from build123d import *

# Parameters (mm, degrees)
SKETCH1_R           = 56.515
BOSS_EXTRUDE1_DEPTH = 19.05


with BuildPart() as part:
    # Sketch1 → Boss-Extrude1 (new body)
    # profile 1 of 6: a face of its own
    with BuildSketch(Plane.XY):
        Polygon((-263.964543073, 0), (-131.982271537, 228.6), (0, 0), align=None)
        with Locations(Location((-131.982271537, 76.2, 0), (0, 0, 180))):
            Circle(SKETCH1_R, mode=Mode.SUBTRACT)
    # profile 2 of 6: a face of its own
    with BuildSketch(Plane.XY):
        Polygon((131.982271537, 228.6), (0, 0), (-131.982271537, 228.6), align=None)
        with Locations(Location((0, 152.4, 0), (0, 0, 180))):
            Circle(SKETCH1_R, mode=Mode.SUBTRACT)
    # profile 3 of 6: a face of its own
    with BuildSketch(Plane.XY):
        Polygon((263.964543073, 0), (0, 0), (131.982271537, 228.6), align=None)
        with Locations(Location((131.982271537, 76.2, 0), (0, 0, 180))):
            Circle(SKETCH1_R, mode=Mode.SUBTRACT)
    # profile 4 of 6: a face of its own
    with BuildSketch(Plane.XY):
        Polygon((131.982271537, -228.6), (0, 0), (263.964543073, 0), align=None)
        with Locations(Location((131.982271537, -76.2, 0), (0, 0, 180))):
            Circle(SKETCH1_R, mode=Mode.SUBTRACT)
    # profile 5 of 6: a face of its own
    with BuildSketch(Plane.XY):
        Polygon((-131.982271537, -228.6), (0, 0), (131.982271537, -228.6), align=None)
        with Locations(Location((0, -152.4, 0), (0, 0, 180))):
            Circle(SKETCH1_R, mode=Mode.SUBTRACT)
    # profile 6 of 6: a face of its own
    with BuildSketch(Plane.XY):
        Polygon((-263.964543073, 0), (0, 0), (-131.982271537, -228.6), align=None)
        with Locations(Location((-131.982271537, -76.2, 0), (0, 0, 180))):
            Circle(SKETCH1_R, mode=Mode.SUBTRACT)
    extrude(amount=BOSS_EXTRUDE1_DEPTH)


solid = part.part
Part model, mm, in its own coordinate system. Coordinates: 2 decimals unless noted, no trailing zeros. Order: outer loops, then holes, each group sorted by start corner. A loop starts at its lowest first (then second) coordinate and runs counter-clockwise, first axis right, second up. Notation, with made-up numbers: M 20.5,61 L 38.5,61 A20 cw 38.5,84 Z; hole C 0,3 d11. An arc over 180 degrees is marked long. Use a Markdown table: item, result.
(1) Cut at A-A on x = 0. Write the cut outline in (y, z) (3 decimals).
A:
| item | result |
|---|---|
| outline | M -228.6,0 L -208.915,0 L -208.915,19.05 L -228.6,19.05 Z; M -95.885,0 L 95.885,0 L 95.885,19.05 L -95.885,19.05 Z; M 208.915,0 L 228.6,0 L 228.6,19.05 L 208.915,19.05 Z |
(2) Cut at C-C on y = 83. Write the cut outline in (x, z).
A:
| item | result |
|---|---|
| outline | M -216.04,0 L -188.09,0 L -188.09,19.05 L -216.04,19.05 Z; M -75.88,0 L 75.88,0 L 75.88,19.05 L -75.88,19.05 Z; M 188.09,0 L 216.04,0 L 216.04,19.05 L 188.09,19.05 Z |
(3) Pull direction Y, two halves, no side cores. Call faces 1 (the flat face through (-2, 228.6, 9)), 2 (the cylindrical face through (12.25, 207.57, 9.39)), 3 (the flat face through (4, 3, 19.05)): released by +Y, released by -Y, zero draft, split by the parting line, or undercut.
A:
| item | result |
|---|---|
| face 1 | released by +Y |
| face 2 | undercut |
| face 3 | zero draft |
(4) Probe L1, parallel to Y at x = 0, z = 13 (3 decimals); L2, parallel to X at y = 93, z = 13; L3, parallel to X at y = -93.5, z = 7.5. List the from-to ranges inside material, lowest first.
A:
| item | result |
|---|---|
| L1 | y = -228.6 to -208.915, -95.885 to 95.885, 208.915 to 228.6 |
| L2 | x = -210.27 to -185.94, -78.02 to 78.02, 185.94 to 210.27 |
| L3 | x = -209.98 to -185.78, -78.18 to 78.18, 185.78 to 209.98 |
(5) Cut at B-B on z = 11. Write the cut outline in (x, y) (3 decimals), then the cut area to 3 significant figures.
A:
| item | result |
|---|---|
| outline | M -263.965,0 L -131.982,-228.6 L 131.982,-228.6 L 263.965,0 L 131.982,228.6 L -131.982,228.6 Z; hole C -131.982,-76.2 d113.03; hole C -131.982,76.2 d113.03; hole C 0,-152.4 d113.03; hole C 0,152.4 d113.03; hole C 131.982,-76.2 d113.03; hole C 131.982,76.2 d113.03 |
| area | 121,000 mm^2 |
(6) Flat gauge pins, fed straight in: pin 1 (8 mm diameter, centred on y = -166.5, z = 6, fed in from -X); pin 2 (2 mm diameter, centred on y = -88, z = 8.5, fed in from -X); pin 3 (1 mm diameter, centred on x = -144, z = 14, fed in from +Y). Where does each tip first touch, or does it go through?
A:
| item | result |
|---|---|
| pin 1 | stops at x = -170.15 |
| pin 2 | stops at x = -213.74 |
| pin 3 | stops at y = 208.65 |
(7) Cut at D-D on y = -152.4. Write the cut outline in (x, z) (3 decimals).
A:
| item | result |
|---|---|
| outline | M -175.976,0 L -56.515,0 L -56.515,19.05 L -175.976,19.05 Z; M 56.515,0 L 175.976,0 L 175.976,19.05 L 56.515,19.05 Z |
